Autodesk Inventor part; units mm, degrees
ref_plane "XZ Plane" through (0, 0, 0) normal (0, 1, 0) x (-1, 0, 0)
sketch "__1" plane through (0, 0, 0) normal (0, 1, 0) x (-1, 0, 0)
  arc A0 (14.1421, -5) -> (14.1421, 5) centre (0, 0) ccw
  line L0 (14.1421, 5) -> (6.5997, 26.3333)
  arc A1 (6.5997, 26.3333) -> (-6.5997, 26.3333) centre (0, 24) ccw
  line L1 (-6.5997, 26.3333) -> (-14.1421, 5)
  arc A2 (-14.1421, 5) -> (-14.1421, -5) centre (0, 0) ccw
  line L2 (-14.1421, -5) -> (-6.5997, -26.3333)
  arc A3 (-6.5997, -26.3333) -> (6.5997, -26.3333) centre (0, -24) ccw
  line L3 (6.5997, -26.3333) -> (14.1421, -5)
  arc A4 (3.25, -23) -> (-3.25, -23) centre (0, -23) ccw
  line L4 (-3.25, -23) -> (-3.25, -25)
  arc A5 (-3.25, -25) -> (3.25, -25) centre (0, -25) ccw
  line L5 (3.25, -25) -> (3.25, -23)
  line L6 (3.25, 23) -> (3.25, 25)
  arc A6 (3.25, 25) -> (-3.25, 25) centre (0, 25) ccw
  line L7 (-3.25, 25) -> (-3.25, 23)
  arc A7 (-3.25, 23) -> (3.25, 23) centre (0, 23) ccw
extrude "Extrusion1" add sketch "__1" along normal blind 2.5
sketch "__2" plane through (0, 0, 0) normal (0, 0, 1) x (1, 0, 0)
  line L0 (0, 2.5) -> (0, 26)
  line L1 (0, 11.9406) -> (3.3235, 13.8594)
  line L2 (3.3235, 13.8594) -> (3.3235, 25.3235)
  line L3 (3.3235, 25.3235) -> (4, 26)
  line L4 (4, 26) -> (15, 26)
  line L5 (15, 26) -> (15, 22.5)
  line L6 (15, 22.5) -> (13.75, 22.5)
  arc A0 (13.75, 22.5) -> (12.5, 21.25) centre (13.75, 21.25) ccw
  line L7 (12.5, 21.25) -> (12.5, 4.25)
  arc A1 (12.5, 4.25) -> (13.75, 3) centre (13.75, 4.25) ccw
  line L8 (13.75, 3) -> (15, 3)
  line L9 (15, 3) -> (15, 2.5)
  line L10 (15, 2.5) -> (0, 2.5)
  line L11 (0, 2.5) -> (0, 11.9406)
revolve "Revolution1" add sketch "__2" angle 360 about axis through (0, 2.5, 0) along (0, -1, 0)
thread "Thread1"
ref_plane "Arbeitsebene1" through (0, 0, 24) normal (0, 0, 1) x (1, 0, 0)
ref_plane "Arbeitsebene2" through (0, 0, -24) normal (0, 0, 1) x (1, 0, 0)
properties part number "NHF19-3026-M8"
Geometry check sheet. Reference: the model listing, model coordinates, mm. A direction names the side the tool comes from. Give positions to 0.01 mm unless a question says otherwise; leave off trailing zeros. Loops run counter-clockwise (first coordinate to the right, second up) from the corner with the lowest first, then second, coordinate; pieces in that order, holes last. Notation, with made-up numbers: (-38, 10.5) -> (15, 10.5) arc R17 cw to (15, 32.5) -> close; hole circle Ø1 at (41.5, 75.25). An arc over 180 degrees is marked (long way). Answer in a Markdown table with one row per item. Add a question column.
1) Cross-section at A-A on y = 19.5. Record the boundary of the cut face in (x, z), and give its area (3 significant figures).
2) Set-up check for faces 1 (the face through (0, 0, 0)), 2 (the face through (4.4, 22.5, -13.3)), 3 (the face through (0.07, 1.23, -19.75)), 4 (the face through (3.07, 19.67, 1.27)): record each of +Z, -Z, +X, -X, +Y, -Y from which the full face is reachable in a straight line by a thin tool's end or side.
3) Gauge pin test, flat ends, axial feed: P1, Ø8.5, axis at x = 0, z = 0, coming from the -Y side; P2, Ø1, axis at y = 1.5, z = -24, coming from the +X side; P3, Ø0.6, axis at y = 1.5, z = 23.5, coming from the -X side; P4, Ø12, axis at x = -9.5, y = 18, coming from the +Z side. Record the tip position at first contact, or that the pin passes through.
4) Draft check along X on faces 5 (the face through (3.25, 1, -24)), 6 (the face through (0, 1, -31)), 7 (the face through (-10.318, 1.232, -15.816)). Enter one of: pulls with the +X half, pulls with the -X half, needs draft (parallel to the pull), parting line crosses it, or undercut.
5) Material ranges on probe 1 along Z at (x, y) = (0, 18.75); probe 2 along Y at (x, z) = (7.25, -21); probe 3 along Z at (x, y) = (-1.5, 18.75), recorded low to high. Write a range as from..to.
6) Cross-section at B-B on y = 6.75. Record the boundary of the cut face in (x, z).
Outcome:
| question | item | result |
|---|---|---|
| 1 | outline | circle Ø25 at (0, 0); hole circle Ø6.65 at (0, 0) |
| 1 | area | 456 mm^2 |
| 2 | face 1 | +Z, -Z, +X, -X, -Y |
| 2 | face 2 | none |
| 2 | face 3 | +Y, -Y |
| 2 | face 4 | +Y |
| 3 | P1 | stops at y = 0 |
| 3 | P2 | stops at x = 7.6 |
| 3 | P3 | stops at x = -7.71 |
| 3 | P4 | stops at z = 13.94 |
| 4 | face 5 | undercut |
| 4 | face 6 | parting line crosses it |
| 4 | face 7 | pulls with the -X half |
| 5 | probe 1 | z = -12.5..-3.32, 3.32..12.5 |
| 5 | probe 2 | y = 0..2.5 |
| 5 | probe 3 | z = -12.41..-2.97, 2.97..12.41 |
| 6 | outline | circle Ø25 at (0, 0) |
